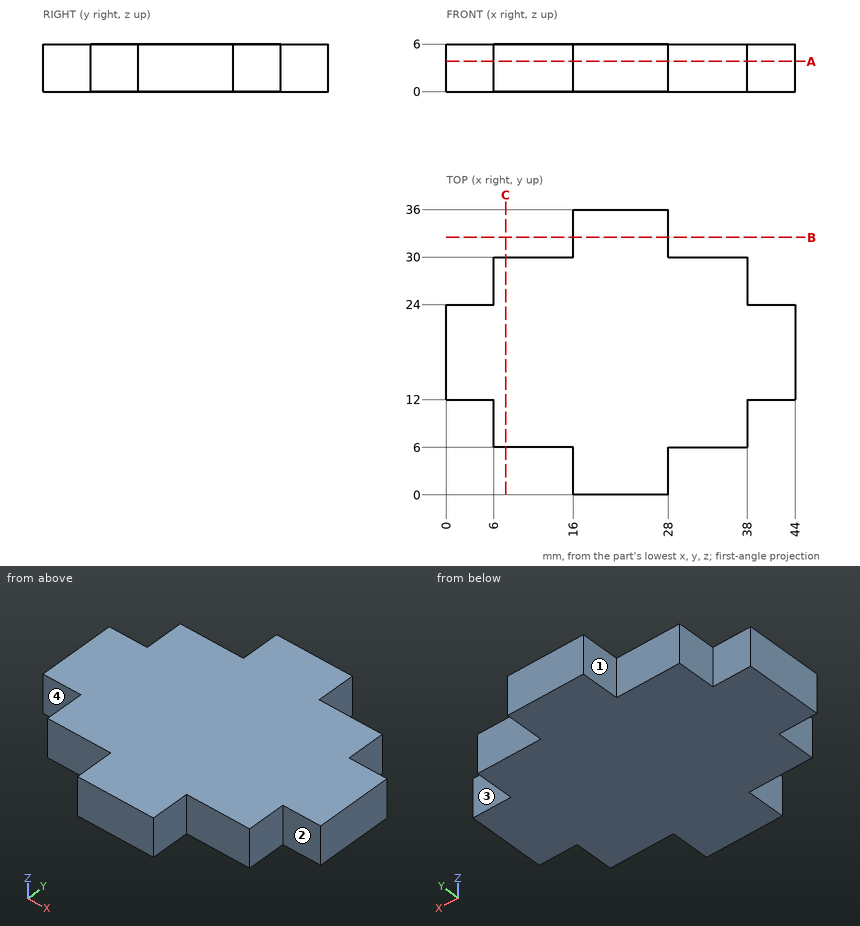
Input: dimensioned drawing with shaded views. Units: mm. Origin: part minimum x, y, z. A direction names the side the tool comes from. Round coordinates to 2 decimals unless told otherwise and drop trailing zeros. Loops run counter-clockwise (first coordinate to the right, second up) from the corner with the lowest first, then second, coordinate; pieces in that order, holes last.
1) Section query C-C on x = 7.5. Return the cut outline in (y, z), plus the area to 3 significant figures.
Ans:
outline: (6, 0) - (30, 0) - (30, 6) - (6, 6) - close
area: 144 mm2
2) Set-up query: the marked faces 1, 2, 3 and 4. Return all of +Z, -Z, +X, -X, +Y, -Y with unobstructed straight access to the full face (end or side cutting, diameter ignored); none if empty.
Ans:
face 1: +Z, -Z, -X, +Y
face 2: +Z, -Z, +X, -Y
face 3: +Z, -Z, +X, +Y
face 4: +Z, -Z, -X, -Y
3) Section query B-B on y = 32.5. Return the cut outline in (x, z).
Ans:
outline: (16, 0) - (28, 0) - (28, 6) - (16, 6) - close
4) Section query A-A on z = 3.8. Return the cut outline in (x, y).
Ans:
outline: (0, 12) - (6, 12) - (6, 6) - (16, 6) - (16, 0) - (28, 0) - (28, 6) - (38, 6) - (38, 12) - (44, 12) - (44, 24) - (38, 24) - (38, 30) - (28, 30) - (28, 36) - (16, 36) - (16, 30) - (6, 30) - (6, 24) - (0, 24) - close
5) Material intervals for line 1 (X direction, y = 5, z = 4.15); line 2 (X direction, y = 11.5, z = 0.95); line 3 (Y direction, x = 34.5, z = 3.75), sorted ascending.
Ans:
line 1: x = 16 to 28
line 2: x = 6 to 38
line 3: y = 6 to 30
6) Pin query (flat end, axial travel): pin 1 (1.8 mm diameter, centred on x = 33, z = 2.5, fed in from -Y); pin 2 (1.8 mm diameter, centred on y = 31.5, z = 2.5, fed in from +X); pin 3 (10 mm diameter, centred on x = 36.5, y = 20.5, fed in from -Z); pin 4 (1.8 mm diameter, centred on y = 28.5, z = 1.5, fed in from -X). Return the tip coordinate at first contact, or that it passes through.
Ans:
pin 1: stops at y = 6
pin 2: stops at x = 28
pin 3: stops at z = 0
pin 4: stops at x = 6
